```python
from build123d import *

# Parameters (mm, degrees)
F0_W     = 4.7625
F0_H     = 38.1
F2_R     = 4.25
F3_DEPTH = 36.5135
F2_R_2   = 12.7
F4_DEPTH = 3.175
F5_R     = 12.7
F5_R_2   = 4.25
F6_DEPTH = 3.175
F5_R_3   = 4.7625
F7_DEPTH = 36.5135


with BuildPart() as f1:
    # F0 (on Front) → F1 (revolve)
    with BuildSketch(Plane.XZ):
        with BuildLine():
            Line((-12.8016, 41.5925), (-15.875, 41.5925))
            Line((-15.875, 41.5925), (-15.875, 0))
            Line((-15.875, 0), (-4.7625, 0))
            ThreePointArc((-4.7625, 0), (0, 4.7625), (4.7625, 0))
            Line((4.7625, 0), (15.875, 0))
            Line((15.875, 0), (15.875, 38.1))
            Line((15.875, 38.1), (15.875, 41.5925))
            Line((15.875, 41.5925), (12.8016, 41.5925))
            Line((12.8016, 41.5925), (8.255, 33.3375))
            Line((8.255, 33.3375), (-8.255, 33.3375))
            Line((-8.255, 33.3375), (-12.8016, 41.5925))
        make_face()
        with Locations((18.25625, 19.05)):
            Rectangle(F0_W, F0_H)
        with BuildLine():
            ThreePointArc((4.7625, 0), (0, 4.7625), (-4.7625, 0))
            Line((-4.7625, 0), (4.7625, 0))
        make_face()
        Polygon((-15.875, 47.1726955307), (-15.875, 41.5925), (-12.8016, 41.5925), align=None)
        Polygon((15.875, 47.1726955307), (12.8016, 41.5925), (15.875, 41.5925), align=None)
    revolve(axis=Axis((2.38125, 0, 0), (1, 0, 0)))

    # F2 (on face) → F3 (cut, through all)
    with BuildSketch(Plane.YZ.offset(20.6375)):
        Circle(F2_R)
    extrude(amount=-F3_DEPTH, mode=Mode.SUBTRACT)

    # F2 (on face) → F4 (cut)
    with BuildSketch(Plane.YZ.offset(20.6375)):
        Circle(F2_R_2)
        Circle(F2_R, mode=Mode.SUBTRACT)
    extrude(amount=-F4_DEPTH, mode=Mode.SUBTRACT)

    # F5 (on face) → F6 (cut)
    with BuildSketch(Plane(origin=(-15.875, 0, 0), x_dir=(0, -1, 0), z_dir=(-1, 0, 0))):
        Circle(F5_R)
        Circle(F5_R_2, mode=Mode.SUBTRACT)
        Circle(F5_R_2)
    extrude(amount=-F6_DEPTH, mode=Mode.SUBTRACT)

    # F5 (on face) → F7 (cut, through all)
    with BuildSketch(Plane(origin=(-15.875, 0, 0), x_dir=(0, -1, 0), z_dir=(-1, 0, 0))):
        with Locations((0, 20.6375)):
            Circle(F5_R_3)
        with Locations((20.6375, 0)):
            Circle(F5_R_3)
        with Locations((0, -20.6375)):
            Circle(F5_R_3)
        with Locations((-20.6375, 0)):
            Circle(F5_R_3)
    extrude(amount=-F7_DEPTH, mode=Mode.SUBTRACT)


solid = f1.part
```
Check sheet for the modelled part. Datum: model origin and axes. Units: mm. A direction names the side the tool comes from. Round coordinates to 2 decimals unless told otherwise and drop trailing zeros. Answer as a JSON object with one key per item and string values.
1. Gauge pin test, flat ends, axial feed: P1, Ø5.5, axis at y = 20.64, z = 0, coming from the -X side; P2, Ø3, axis at x = -3.5, y = -15.5, coming from the +Z side; P3, Ø3, axis at x = 6, y = 2.5, coming from the +Z side; P4, Ø1.5, axis at x = 9.5, z = 20.5, coming from the +Y side. Record the tip position at first contact, or that the pin passes through.
Reply:
{"P1": "passes through", "P2": "stops at z = 30.26", "P3": "stops at z = 33.32", "P4": "stops at y = 30.83"}
2. Scan lines: line 1 (Z direction, x = 19.9, y = 0) (3 decimals); line 2 (X direction, y = 31, z = -24) (3 decimals); line 3 (X direction, y = -33.5, z = 22) (3 decimals). Record each from-to range of solid material in increasing order.
Reply:
{"line 1": "z = -38.1 to -25.4, -15.875 to -12.7, 12.7 to 15.875, 25.4 to 38.1", "line 2": "x = -15.875 to -11.486, 11.486 to 15.875", "line 3": "x = -15.875 to -11.967, 11.967 to 15.875"}
3. Section check A-A (x = -1.5). State how many separate pieces and enclosed holes the cut face has, plus the area to 3 significant figures.
Reply:
{"separate pieces": "1", "enclosed holes": "5", "area": "3,150 mm²"}
4. Mould release check, pull along Y, two halves, no side actions. Record for faces 1 (the flat face through (-15.875, 10, 10)), 2 (the cylindrical face through (-0.12, -10.01, 31.8)), 3 (the cylindrical face through (2.126, 25.395, 0.209)), 4 (the cylindrical face through (2.13, -25.04, -1.82)): pulls with the +Y half, pulls with the -Y half, needs draft (parallel to the pull), parting line crosses it, or undercut.
Reply:
{"face 1": "needs draft", "face 2": "parting line crosses it", "face 3": "undercut", "face 4": "undercut"}
5. Access from +Z, -Z, +X, -X, +Y, -Y to the whole of each face (thin tool, end or side, straight path). Record for faces 5 (the flat face through (-12.7, -5, 0)), 6 (the flat face through (17.462, 5, 0)), 7 (the cylindrical face through (2.13, 0.62, 25.36)).
Reply:
{"face 5": "-X", "face 6": "+X", "face 7": "+X, -X"}
